Could you check a few things on this drawing? It's one solid part, dimensions in mm from its lowest x, y, z. A direction names the side the tool comes from. Round coordinates to 2 decimals unless told otherwise and drop trailing zeros. Write each loop counter-clockwise with the first axis right and the second up, starting at its lowest first coordinate (ties: lowest second). Pieces come first, ordered by that corner, then holes. Notation, with made-up numbers: (77.5, 12) - (132.5, 12) arc R30 ccw to (132.5, 47) - close; hole circle Ø1 at (-3.5, 89.5). An arc over 180 degrees is marked (long way). Write item = value, one per line. Start each with the question number.
Item 1: Which directions (+Z, -Z, +X, -X, +Y, -Y) give clear straight access to the entire face, cutting with the end or side of a thin tool? Please do the marked faces 4 and 5.
Item 2: If we section it at A-A (z = 24.5): Please give me the cut outline in (x, y), and give its area (3 significant figures).
Item 3: If we section it at B-B (y = 2.7): Please give me the cut outline in (x, z).
Item 4: Thinking about a two-plate mould opening in X: for the marked faces 1, 2 and 3, which applies, pulls with the +X half, pulls with the -X half, needs draft (parallel to the pull), parting line crosses it, or undercut?
Item 5: For P1, Ø6, axis at x = 8.5, z = 5.5, coming from the -Y side; P2, Ø1.2, axis at y = 3, z = 19.5, coming from the -X side; P3, Ø1.2, axis at x = 5, y = 3, coming from the -Z side, each with a flat end and sliding along its axis, tell me the tip position at first contact or that it passes through.
Item 6: If we section it at C-C (x = 8.5): Please give me the cut outline in (y, z), and give its area (3 significant figures).
Item 7: If I drill on line 1 along X through (y, z) = (1.9, 15.25); line 2 along Z through (x, y) = (4, 0.6); line 3 along Y through (x, z) = (4.25, 4), over which ranges is the centre line in solid material (lowest first)? Write a range as [from, to].
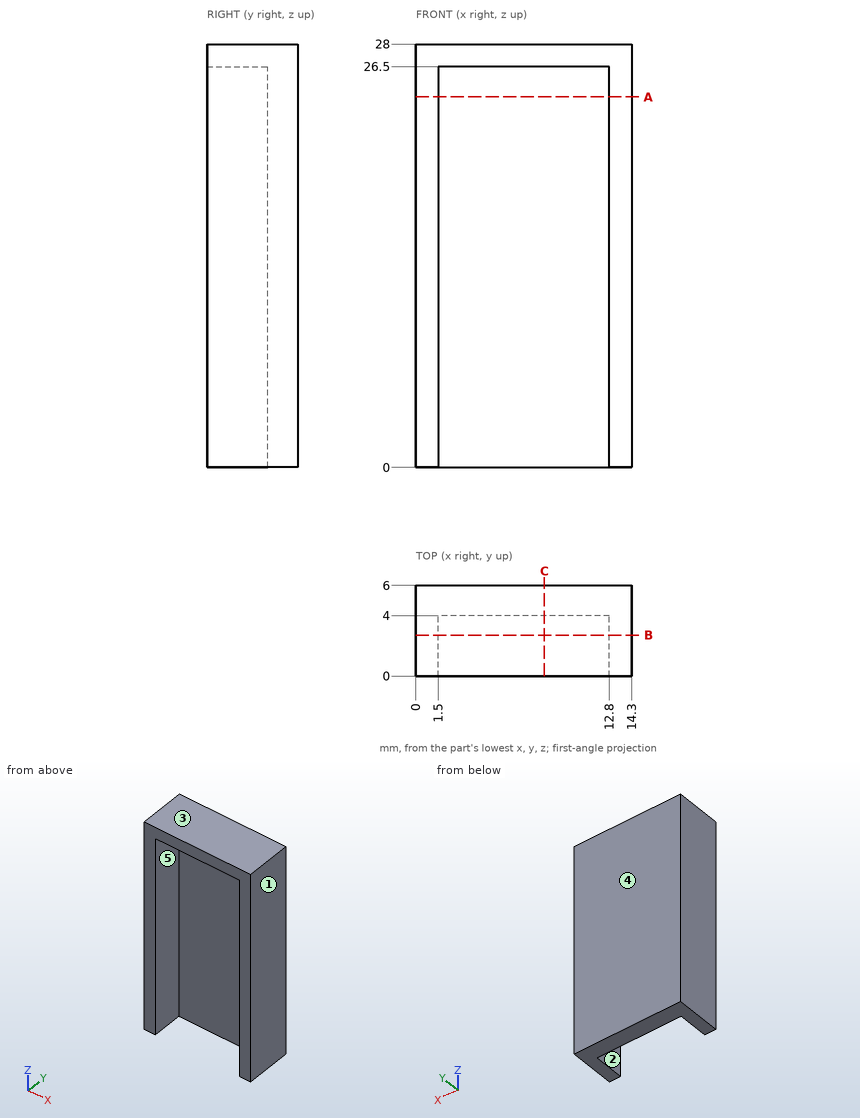
Reply:
q1.face_4 = +Z, -Z, +X, -X, +Y
q1.face_5 = -Z, -Y
q2.outline = (0, 0) - (1.5, 0) - (1.5, 4) - (12.8, 4) - (12.8, 0) - (14.3, 0) - (14.3, 6) - (0, 6) - close
q2.area = 40.6 mm2
q3.outline = (0, 0) - (1.5, 0) - (1.5, 26.5) - (12.8, 26.5) - (12.8, 0) - (14.3, 0) - (14.3, 28) - (0, 28) - close
q4.face_1 = pulls with the +X half
q4.face_2 = undercut
q4.face_3 = needs draft
q5.P1 = 4
q5.P2 = 0
q5.P3 = 26.5
q6.outline = (0, 26.5) - (4, 26.5) - (4, 0) - (6, 0) - (6, 28) - (0, 28) - close
q6.area = 62.0 mm2
q7.line_1 = [0, 1.5], [12.8, 14.3]
q7.line_2 = [26.5, 28]
q7.line_3 = [4, 6]
